```python
from build123d import *

# Parameters (mm, degrees)
BOSS_EXTRUDE1_DEPTH            = 60
CUT_EXTRUDE1_REACH             = 69.704
CUT_EXTRUDE1_END_RADIUS        = 20
SKETCH3_R                      = 2.5
CUT_EXTRUDE1_DIRECTION_2_DEPTH = 68.704354886


with BuildPart() as part:
    # Sketch2 → Boss-Extrude1 (new body)
    with BuildSketch(Plane.XY):
        with BuildLine():
            Line((0, 22.452229299), (0, -27.547770701))
            Line((0, -27.547770701), (-15, -27.547770701))
            Line((-15, -27.547770701), (-15, -17.547770701))
            ThreePointArc((-15, -17.547770701), (-8.228756555, -2.547770701), (-15, 12.452229299))
            Line((-15, 12.452229299), (-15, 22.452229299))
            Line((-15, 22.452229299), (0, 22.452229299))
        make_face()
    extrude(amount=BOSS_EXTRUDE1_DEPTH)

    # Cut-Extrude1: up to this cylinder (the profile starts outside it)
    cut_extrude1_end = Plane(origin=(-28.228756555, -2.547770701, 30), z_dir=(0, 0, -1)) * Cylinder(CUT_EXTRUDE1_END_RADIUS, 210.408, mode=Mode.PRIVATE)
    # Sketch3 → Cut-Extrude1 (cut, up to the surface)
    with BuildSketch(Plane(origin=(0, 0, 0), x_dir=(0, 0, -1), z_dir=(1, 0, 0)), mode=Mode.PRIVATE) as cut_extrude1_sk1:
        with Locations(Location((-15, -2.547770701, 0), (0, 0, 180))):
            Circle(SKETCH3_R)
    cut_extrude1_tool1 = extrude(cut_extrude1_sk1.sketch, amount=-CUT_EXTRUDE1_REACH, mode=Mode.PRIVATE) - cut_extrude1_end
    add(cut_extrude1_tool1.solids().sort_by_distance((0, -2.547771, 15))[0], mode=Mode.SUBTRACT)
    # Sketch3 → Cut-Extrude1 (cut, up to the surface)
    with BuildSketch(Plane(origin=(0, 0, 0), x_dir=(0, 0, -1), z_dir=(1, 0, 0)), mode=Mode.PRIVATE) as cut_extrude1_sk2:
        with Locations(Location((-45, -2.547770701, 0), (0, 0, 180))):
            Circle(SKETCH3_R)
    cut_extrude1_tool2 = extrude(cut_extrude1_sk2.sketch, amount=-CUT_EXTRUDE1_REACH, mode=Mode.PRIVATE) - cut_extrude1_end
    add(cut_extrude1_tool2.solids().sort_by_distance((0, -2.547771, 45))[0], mode=Mode.SUBTRACT)

    # Sketch3 → Cut-Extrude1 direction 2 (cut)
    with BuildSketch(Plane(origin=(0, 0, 0), x_dir=(0, 0, -1), z_dir=(1, 0, 0))):
        with Locations(Location((-15, -2.547770701, 0), (0, 0, 180))):
            Circle(SKETCH3_R)
        with Locations(Location((-45, -2.547770701, 0), (0, 0, 180))):
            Circle(SKETCH3_R)
    extrude(amount=CUT_EXTRUDE1_DIRECTION_2_DEPTH, mode=Mode.SUBTRACT)


solid = part.part
```
The model under review builds one solid part; all positions refer to its coordinate system, in mm. Round coordinates to 2 decimals unless told otherwise and drop trailing zeros. Order: outer loops, then holes, each group sorted by start corner. A loop starts at its lowest first (then second) coordinate and runs counter-clockwise, first axis right, second up. Notation, with made-up numbers: (58, 49) - (115, 49) arc R25 ccw to (115, 76) - close; hole circle Ø4 at (3, 74.25). An arc over 180 degrees is marked (long way). Answer in a Markdown table with one row per item.
(1) Take a section at C-C on y = -15.5. Write out the cut boundary in (x, z), plus the area to 3 significant figures.
Result set:
| item | result |
|---|---|
| outline | (-12.99, 0) - (0, 0) - (0, 60) - (-12.99, 60) - close |
| area | 779 mm2 |
(2) Take a section at A-A on z = 15. Write out the cut boundary in (x, y), plus the area to 3 significant figures.
Result set:
| item | result |
|---|---|
| outline | (-15, -27.55) - (0, -27.55) - (0, -5.05) - (-8.39, -5.05) arc R20 cw to (-15, -17.55) - close; (-15, 12.45) arc R20 cw to (-8.39, -0.05) - (0, -0.05) - (0, 22.45) - (-15, 22.45) - close |
| area | 568 mm2 |
(3) Clearance check with flat-ended pins moving along their axes: P1, Ø1, axis at y = -13.5, z = 50, coming from the -X side; P2, Ø2, axis at y = -6.5, z = 33.5, coming from the -X side. State where each tip first meets the part, or that it passes through.
Result set:
| item | result |
|---|---|
| P1 | stops at x = -11.83 |
| P2 | stops at x = -8.85 |
(4) Take a section at B-B on z = 56.5. Write out the cut boundary in (x, y), plus the area to 3 significant figures.
Result set:
| item | result |
|---|---|
| outline | (-15, -27.55) - (0, -27.55) - (0, 22.45) - (-15, 22.45) - (-15, 12.45) arc R20 cw to (-15, -17.55) - close |
| area | 609 mm2 |
(5) For line 1 (Y direction, x = -6, z = 45); line 2 (Y direction, x = -7, z = 43.5); line 3 (X direction, y = -5, z = 39), list the stretches that pass through material, from the lowest coordinate up. Write a range as from..to.
Result set:
| item | result |
|---|---|
| line 1 | y = -27.55..-5.05, -0.05..22.45 |
| line 2 | y = -27.55..-4.55, -0.55..22.45 |
| line 3 | x = -8.38..0 |
(6) Take a section at D-D on y = 5. Write out the cut boundary in (x, z).
Result set:
| item | result |
|---|---|
| outline | (-9.71, 0) - (0, 0) - (0, 60) - (-9.71, 60) - close |
